For this review, take the finished solid that the model builds, in its own axes (mm). Face numbers are marked on the shaded views. A direction names the side the tool comes from. Round coordinates to 2 decimals unless told otherwise and drop trailing zeros. Write each question's results on one line, items separated by ' | '.
```python
from build123d import *

# Parameters (mm, degrees)
F2_SIZE  = 0.5
F5_DEPTH = 25


with BuildPart() as f1:
    # F0 (on Front) → F1 (revolve)
    with BuildSketch(Plane.XZ):
        Polygon((0, 23), (0, 0), (0, -101), (2.5, -103.5), (2.5, -106), (12.5, -106), (12.5, -105), (12.5, -75), (15, -75), (15, -51), (15, -46), (12.5, -46), (12.5, -6), (11.95, -6), (11.95, -4.7), (12.5, -4.7), (12.5, -1.3), (11.95, -1.3), (11.95, 0), (12.5, 0), (12.5, 24), (11.95, 24), (11.95, 25.3), (12.475, 25.3), (12.475, 28), (2.5, 28), (2.5, 25.5), align=None)
    revolve(axis=Axis((0, 0, -50.5), (0, 0, 1)))

    # F2
    f2_edges = [f1.edges().sort_by_distance(p)[0] for p in [
        (-15, 0, -46),
        (-12.5, 0, -46),
        (-12.5, 0, -75),
        (-15, 0, -75),
        (-12.475, 0, 28),
        (-2.5, 0, -106),
        (-12.5, 0, -106),
    ]]
    chamfer(f2_edges, length=F2_SIZE)

    # F4 (on offset) → F5 (cut)
    with BuildSketch(Plane.XZ.offset(8.5)):
        with BuildLine():
            ThreePointArc((-4, -39.5), (0, -43.5), (4, -39.5))
            Line((4, -39.5), (4, -12.5))
            ThreePointArc((4, -12.5), (0, -8.5), (-4, -12.5))
            Line((-4, -12.5), (-4, -39.5))
        make_face()
        with BuildLine():
            Line((4, -98.5), (4, -81.5))
            ThreePointArc((4, -81.5), (0, -77.5), (-4, -81.5))
            Line((-4, -81.5), (-4, -98.5))
            ThreePointArc((-4, -98.5), (0, -102.5), (4, -98.5))
        make_face()
    extrude(amount=F5_DEPTH, mode=Mode.SUBTRACT)


solid = f1.part
```
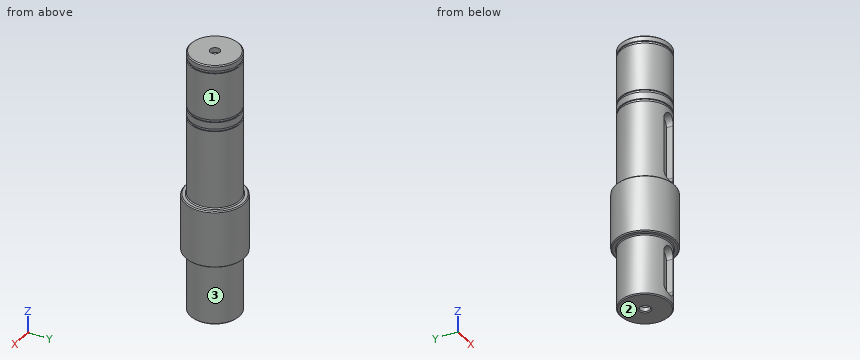
1. Consider section A-A (y = -10.25). Give the number of separate pieces and of enclosed holes in the cut face, plus the area to 3 significant figures.
Values found:
separate pieces: 1 | enclosed holes: 2 | area: 1,680 mm2
2. To check wall thickness, follow probe 1 along Y at (x, z) = (0, 27) (3 decimals); probe 2 along Z at (x, y) = (-9.5, -8); probe 3 along X at (y, z) = (-0.5, -34.5). State the ranges of each line that lie inside material, in increasing order.
Values found:
probe 1: y = -12.475 to -2.5, 2.5 to 12.475 | probe 2: z = -105.58 to -6, -4.7 to -1.3, 0 to 24, 25.3 to 27.56 | probe 3: x = -12.49 to 12.49
3. Tool access review of the marked faces 1, 2 and 3: name each direction out of +Z, -Z, +X, -X, +Y, -Y from which nothing blocks a thin tool from reaching the whole face with its end or side.
Values found:
face 1: +Z | face 2: -Z, +X, -X, +Y, -Y | face 3: -Z
4. For pin 1 (8 mm diameter, centred on x = -0.5, z = 2.5, fed in from -Y); pin 2 (4.5 mm diameter, centred on x = 0, y = 0, fed in from -Z); pin 3 (1.5 mm diameter, centred on x = -12, y = 11.5, fed in from +Z); pin 4 (1.7 mm diameter, centred on y = -9.5, z = -30.5, fed in from +X), all flat-tipped, find the tip position at first contact; note any pin that passes through.
Values found:
pin 1: stops at y = -12.5 | pin 2: stops at z = -103.25 | pin 3: passes through | pin 4: stops at x = 9.02
